Geometry check sheet. Reference: drawing and pictorial views, mm from the part's lowest x, y, z. A direction names the side the tool comes from. Round coordinates to 2 decimals unless told otherwise and drop trailing zeros. Loops run counter-clockwise (first coordinate to the right, second up) from the corner with the lowest first, then second, coordinate; pieces in that order, holes last. Notation, with made-up numbers: (3, 62) - (48, 62) arc R23 cw to (48, 100) - close; hole circle Ø7 at (17, 41). An arc over 180 degrees is marked (long way). Answer as CSV lines item,"result". Start each with the question number.
1) Cross-section at A-A on x = 16.5. Record the boundary of the cut face in (y, z), and give its area (3 significant figures).
2) Thickness scan on line 1 along Y through (x, z) = (14, 4.5); line 2 along Z through (x, y) = (7.25, 6.25). Record the ranges inside material, lowest first.
3) Depth check by flat-ended pin: P1, Ø1, axis at x = 16, y = 13, coming from the +Z side. Enter the tip coordinate at first touch or a pass-through.
4) Draft check along Y on the marked faces 3, 4 and 5. Enter one of: released by +Y, released by -Y, zero draft, split by the parting line, or undercut.
5) Access from +Z, -Z, +X, -X, +Y, -Y to the whole of each face (thin tool, end or side, straight path). Record for the marked faces 1 and 2.
6) Cross-section at B-B on z = 3. Record the boundary of the cut face in (x, y), and give its area (3 significant figures).
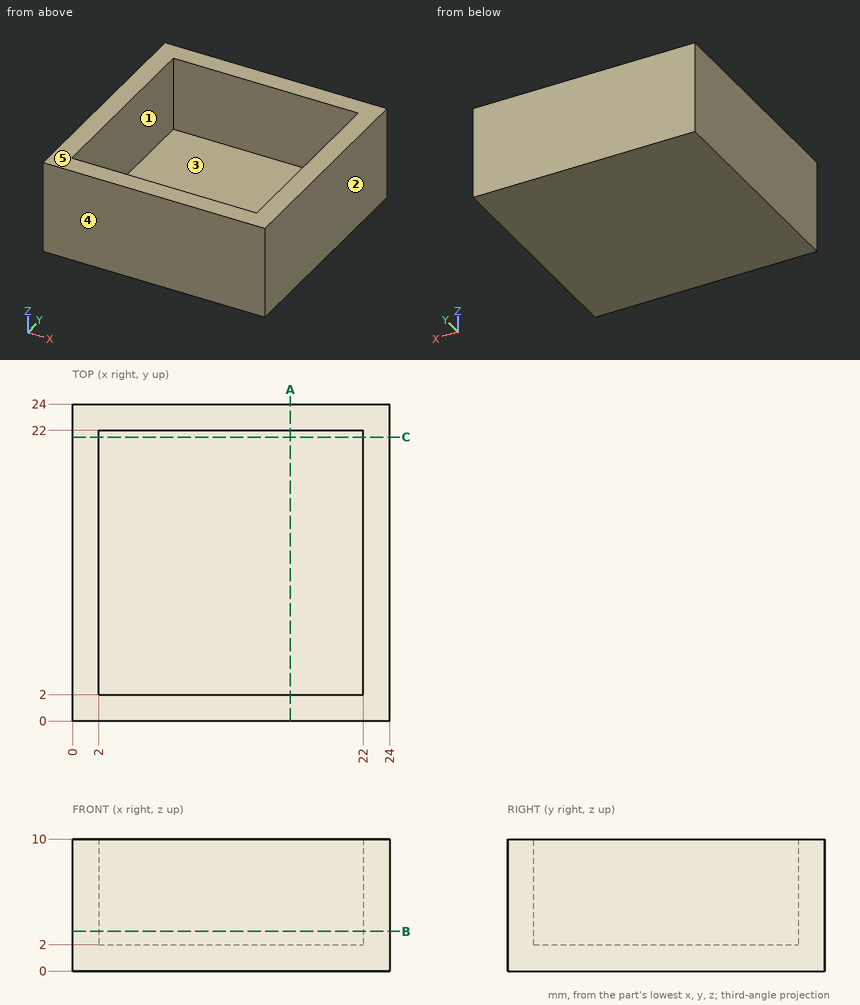
Answer block:
1,outline,"(0, 0) - (24, 0) - (24, 10) - (22, 10) - (22, 2) - (2, 2) - (2, 10) - (0, 10) - close"
1,area,"80.0 mm^2"
2,line 1,"y = 0 to 2, 22 to 24"
2,line 2,"z = 0 to 2"
3,P1,"stops at z = 2"
4,face 3,"undercut"
4,face 4,"released by -Y"
4,face 5,"zero draft"
5,face 1,"+Z"
5,face 2,"+Z, -Z, +X, +Y, -Y"
6,outline,"(0, 0) - (24, 0) - (24, 24) - (0, 24) - close; hole (2, 2) - (22, 2) - (22, 22) - (2, 22) - close"
6,area,"176 mm^2"
